Model file for the job. Use its own axes, mm. Face numbers are marked on the shaded views. Give positions to 0.01 mm unless a question says otherwise; leave off trailing zeros. Loops run counter-clockwise (first coordinate to the right, second up) from the corner with the lowest first, then second, coordinate; pieces in that order, holes last. Notation, with made-up numbers: M 45,25 L 88,25 A22 cw 88,52 Z; hole C 63,52 d2. An arc over 180 degrees is marked long. Answer in a Markdown table with one row per item.
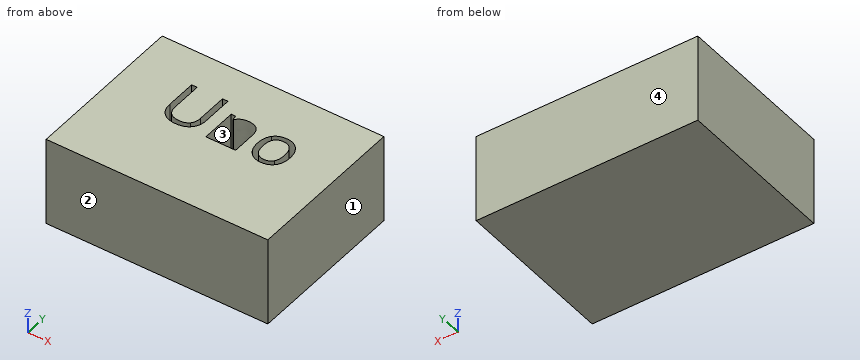
```python
from build123d import *

# Parameters (mm, degrees)
F0_W     = 75
F0_H     = 55
F1_DEPTH = 30
F3_DEPTH = 25


with BuildPart() as f1:
    # F0 (on Top) → F1 (new body)
    with BuildSketch(Plane.XY):
        with Locations((-1.7472282052, 5.8279882101)):
            Rectangle(F0_W, F0_H)
    extrude(amount=F1_DEPTH)

    # F2 (on face) → F3 (cut)
    with BuildSketch(Plane.XY.offset(30)):
        with BuildLine():
            Line((-4.0867042615, 16.8077548728), (-4.0867042615, 4.7675450332))
            Line((-4.0867042615, 4.7675450332), (-2.2622169894, 4.7675450332))
            Line((-2.2622169894, 4.7675450332), (-2.2622169894, 11.0847003856))
            add(Edge.make_bspline(
                [(-1.3833695559, 14.4577168355), (-2.2622169894, 13.4364961177), (-2.2622169894, 11.0847003856)],
                knots=[0, 0, 0, 1, 1, 1], degree=2))
            add(Edge.make_bspline(
                [(1.3832421649, 15.4789375533), (-0.5045221224, 15.4789375533), (-1.3833695559, 14.4577168355)],
                knots=[0, 0, 0, 1, 1, 1], degree=2))
            add(Edge.make_bspline(
                [(3.4836875311, 14.7530095732), (2.8140057867, 15.4789375533), (1.3832421649, 15.4789375533)],
                knots=[0, 0, 0, 1, 1, 1], degree=2))
            add(Edge.make_bspline(
                [(4.1533692754, 12.5576486842), (4.1533692754, 14.0270815931), (3.4836875311, 14.7530095732)],
                knots=[0, 0, 0, 1, 1, 1], degree=2))
            Line((4.1533692754, 12.5576486842), (4.1533692754, 4.7675450332))
            Line((4.1533692754, 4.7675450332), (5.9778565475, 4.7675450332))
            Line((5.9778565475, 4.7675450332), (5.9778565475, 12.6209256994))
            add(Edge.make_bspline(
                [(4.8792972555, 15.9798805904), (5.9778565475, 14.9305367547), (5.9778565475, 12.6209256994)],
                knots=[0, 0, 0, 1, 1, 1], degree=2))
            add(Edge.make_bspline(
                [(1.6047117181, 17.029224426), (3.7807379636, 17.029224426), (4.8792972555, 15.9798805904)],
                knots=[0, 0, 0, 1, 1, 1], degree=2))
            add(Edge.make_bspline(
                [(-0.6468954066, 16.5388275581), (0.363779142, 17.029224426), (1.6047117181, 17.029224426)],
                knots=[0, 0, 0, 1, 1, 1], degree=2))
            add(Edge.make_bspline(
                [(-2.2200323126, 15.1590370875), (-1.6575699552, 16.0484306902), (-0.6468954066, 16.5388275581)],
                knots=[0, 0, 0, 1, 1, 1], degree=2))
            Line((-2.2200323126, 15.1590370875), (-2.307917056, 15.1590370875))
            Line((-2.307917056, 15.1590370875), (-2.6032097937, 16.8077548728))
            Line((-2.6032097937, 16.8077548728), (-4.0867042615, 16.8077548728))
        make_face()
        with BuildLine():
            add(Edge.make_bspline(
                [(-12.2786519386, 4.7675450332), (-13.1925449458, 4.54607548), (-14.2813344906, 4.54607548)],
                knots=[0.6245807712, 0.6245807712, 0.6245807712, 1, 1, 1], degree=2))
            Line((-12.2786519386, 4.7675450332), (-16.2668224103, 4.7675450332))
            add(Edge.make_bspline(
                [(-14.2813344906, 4.54607548), (-15.3658863063, 4.54607548), (-16.2668224103, 4.7675450332)],
                knots=[0, 0, 0, 0.3739580419, 0.3739580419, 0.3739580419], degree=2))
        make_face()
        with BuildLine():
            Line((-16.2668224103, 4.7675450332), (-12.2786519386, 4.7675450332))
            add(Edge.make_bspline(
                [(-9.7218740054, 6.1174546912), (-10.7582183658, 5.1360014515), (-12.2786519386, 4.7675450332)],
                knots=[0, 0, 0, 0.6245807712, 0.6245807712, 0.6245807712], degree=2))
            add(Edge.make_bspline(
                [(-8.0626100508, 10.4378686745), (-8.0626100508, 7.6888339023), (-9.7218740054, 6.1174546912)],
                knots=[0, 0, 0, 1, 1, 1], degree=2))
            Line((-8.0626100508, 10.4378686745), (-8.0626100508, 20.8293607287))
            Line((-8.0626100508, 20.8293607287), (-9.9292819997, 20.8293607287))
            Line((-9.9292819997, 20.8293607287), (-9.9292819997, 10.3710762695))
            add(Edge.make_bspline(
                [(-11.0278412916, 7.2669871342), (-9.9292819997, 8.3497271724), (-9.9292819997, 10.3710762695)],
                knots=[0, 0, 0, 1, 1, 1], degree=2))
            add(Edge.make_bspline(
                [(-14.1582958499, 6.1842470961), (-12.1264005835, 6.1842470961), (-11.0278412916, 7.2669871342)],
                knots=[0, 0, 0, 1, 1, 1], degree=2))
            add(Edge.make_bspline(
                [(-17.3871813207, 7.2617140496), (-16.2886220288, 6.1842470961), (-14.1582958499, 6.1842470961)],
                knots=[0, 0, 0, 1, 1, 1], degree=2))
            add(Edge.make_bspline(
                [(-18.4857406127, 10.3499839311), (-18.4857406127, 8.3391810032), (-17.3871813207, 7.2617140496)],
                knots=[0, 0, 0, 1, 1, 1], degree=2))
            Line((-18.4857406127, 10.3499839311), (-18.4857406127, 20.8293607287))
            Line((-18.4857406127, 20.8293607287), (-20.3559279512, 20.8293607287))
            Line((-20.3559279512, 20.8293607287), (-20.3559279512, 10.4800533513))
            add(Edge.make_bspline(
                [(-18.7687294863, 6.1297585552), (-20.3559279512, 7.7134416305), (-20.3559279512, 10.4800533513)],
                knots=[0, 0, 0, 1, 1, 1], degree=2))
            add(Edge.make_bspline(
                [(-16.2668224103, 4.7675450332), (-17.7750766513, 5.1383065018), (-18.7687294863, 6.1297585552)],
                knots=[0.3739580419, 0.3739580419, 0.3739580419, 1, 1, 1], degree=2))
        make_face()
        with BuildLine():
            add(Edge.make_bspline(
                [(12.8943034011, 4.7675450332), (12.2413601129, 4.9561574078), (11.6657571374, 5.3053996626)],
                knots=[0.5400617249, 0.5400617249, 0.5400617249, 1, 1, 1], degree=2))
            Line((12.8943034011, 4.7675450332), (16.2966207559, 4.7675450332))
            add(Edge.make_bspline(
                [(18.6315018956, 6.2000663499), (17.691967628, 5.1513098305), (16.2966207559, 4.7675450332)],
                knots=[0, 0, 0, 0.6340763655, 0.6340763655, 0.6340763655], degree=2))
            add(Edge.make_bspline(
                [(20.1132386686, 10.7999538171), (20.1132386686, 7.8540572199), (18.6315018956, 6.2000663499)],
                knots=[0, 0, 0, 1, 1, 1], degree=2))
            add(Edge.make_bspline(
                [(18.6244711162, 15.3471104382), (20.1132386686, 13.6649964504), (20.1132386686, 10.7999538171)],
                knots=[0, 0, 0, 1, 1, 1], degree=2))
            add(Edge.make_bspline(
                [(14.6116537346, 17.029224426), (17.1357035637, 17.029224426), (18.6244711162, 15.3471104382)],
                knots=[0, 0, 0, 1, 1, 1], degree=2))
            add(Edge.make_bspline(
                [(10.5232554737, 15.3857797253), (11.9962037724, 17.029224426), (14.6116537346, 17.029224426)],
                knots=[0, 0, 0, 1, 1, 1], degree=2))
            add(Edge.make_bspline(
                [(9.0503071751, 10.7999538171), (9.0503071751, 13.7423350246), (10.5232554737, 15.3857797253)],
                knots=[0, 0, 0, 1, 1, 1], degree=2))
            add(Edge.make_bspline(
                [(9.7322927836, 7.481425908), (9.0503071751, 8.8981279709), (9.0503071751, 10.7999538171)],
                knots=[0, 0, 0, 1, 1, 1], degree=2))
            add(Edge.make_bspline(
                [(11.6657571374, 5.3053996626), (10.414278392, 6.0647238452), (9.7322927836, 7.481425908)],
                knots=[0, 0, 0, 1, 1, 1], degree=2))
        make_face()
        with BuildLine():
            add(Edge.make_bspline(
                [(10.9415868521, 10.7999538171), (10.9415868521, 8.4903427617), (11.8643766573, 7.282806388)],
                knots=[0, 0, 0, 1, 1, 1], degree=2))
            add(Edge.make_bspline(
                [(11.8538304881, 14.3030396872), (10.9415868521, 13.1271418211), (10.9415868521, 10.7999538171)],
                knots=[0, 0, 0, 1, 1, 1], degree=2))
            add(Edge.make_bspline(
                [(14.5554074988, 15.4789375533), (12.7660741242, 15.4789375533), (11.8538304881, 14.3030396872)],
                knots=[0, 0, 0, 1, 1, 1], degree=2))
            add(Edge.make_bspline(
                [(17.2974114915, 14.2872204334), (16.3693486017, 15.4789375533), (14.5554074988, 15.4789375533)],
                knots=[0, 0, 0, 1, 1, 1], degree=2))
            add(Edge.make_bspline(
                [(18.2254743813, 10.7999538171), (18.2254743813, 13.0955033135), (17.2974114915, 14.2872204334)],
                knots=[0, 0, 0, 1, 1, 1], degree=2))
            add(Edge.make_bspline(
                [(17.2974114915, 7.2775333034), (18.2254743813, 8.4797965925), (18.2254743813, 10.7999538171)],
                knots=[0, 0, 0, 1, 1, 1], degree=2))
            add(Edge.make_bspline(
                [(14.5764998373, 6.0752700144), (16.3693486017, 6.0752700144), (17.2974114915, 7.2775333034)],
                knots=[0, 0, 0, 1, 1, 1], degree=2))
            add(Edge.make_bspline(
                [(11.8643766573, 7.282806388), (12.7871664626, 6.0752700144), (14.5764998373, 6.0752700144)],
                knots=[0, 0, 0, 1, 1, 1], degree=2))
        make_face(mode=Mode.SUBTRACT)
        with BuildLine():
            Line((16.2966207559, 4.7675450332), (12.8943034011, 4.7675450332))
            add(Edge.make_bspline(
                [(14.5343151604, 4.54607548), (13.6609925365, 4.54607548), (12.8943034011, 4.7675450332)],
                knots=[0, 0, 0, 0.5400617249, 0.5400617249, 0.5400617249], degree=2))
            add(Edge.make_bspline(
                [(16.2966207559, 4.7675450332), (15.4913701164, 4.54607548), (14.5343151604, 4.54607548)],
                knots=[0.6340763655, 0.6340763655, 0.6340763655, 1, 1, 1], degree=2))
        make_face()
        with BuildLine():
            Line((-2.2622169894, 11.0847003856), (-2.2622169894, 4.7675450332))
            Line((-2.2622169894, 4.7675450332), (4.1533692754, 4.7675450332))
            Line((4.1533692754, 4.7675450332), (4.1533692754, 12.5576486842))
            add(Edge.make_bspline(
                [(4.1533692754, 12.5576486842), (4.1533692754, 14.0270815931), (3.4836875311, 14.7530095732)],
                knots=[0, 0, 0, 1, 1, 1], degree=2))
            add(Edge.make_bspline(
                [(3.4836875311, 14.7530095732), (2.8140057867, 15.4789375533), (1.3832421649, 15.4789375533)],
                knots=[0, 0, 0, 1, 1, 1], degree=2))
            add(Edge.make_bspline(
                [(1.3832421649, 15.4789375533), (-0.5045221224, 15.4789375533), (-1.3833695559, 14.4577168355)],
                knots=[0, 0, 0, 1, 1, 1], degree=2))
            add(Edge.make_bspline(
                [(-1.3833695559, 14.4577168355), (-2.2622169894, 13.4364961177), (-2.2622169894, 11.0847003856)],
                knots=[0, 0, 0, 1, 1, 1], degree=2))
        make_face()
    extrude(amount=-F3_DEPTH, mode=Mode.SUBTRACT)


solid = f1.part
```
Q1. Saw through at B-B (y = 19.5). Give the cut face in (x, z).
Reported:
| item | result |
|---|---|
| outline | M -39.25,0 L 35.75,0 L 35.75,30 L -8.06,30 L -8.06,5 L -9.93,5 L -9.93,30 L -18.49,30 L -18.49,5 L -20.36,5 L -20.36,30 L -39.25,30 Z |
Q2. Saw through at A-A (z = 13.5). Give the number of separate pieces and of enclosed holes in the cut face, and give its area (3 significant figures).
Reported:
| item | result |
|---|---|
| separate pieces | 2 |
| enclosed holes | 3 |
| area | 3,880 mm² |
Q3. Probe probe 1 along Y at (x, z) = (17, 6); probe 2 along Y at (x, z) = (16, 16); probe 3 along Y at (x, z) = (-4, 21). List the from-to ranges inside material, lowest first.
Reported:
| item | result |
|---|---|
| probe 1 | -21.67 to 5.02, 6.94 to 14.62, 16.56 to 33.33 |
| probe 2 | -21.67 to 4.69, 6.31 to 15.24, 16.89 to 33.33 |
| probe 3 | -21.67 to 4.77, 16.81 to 33.33 |
Q4. Mould opens along Y. For the marked faces 1, 2, 3 and 4 say: released by +Y, released by -Y, zero draft, split by the parting line, or undercut.
Reported:
| item | result |
|---|---|
| face 1 | zero draft |
| face 2 | released by -Y |
| face 3 | undercut |
| face 4 | released by +Y |
Q5. Drop a flat-ended pin along its axis: pin 1 (5 mm diameter, centred on x = -1.5, y = 8.5, fed in from +Z). Give the stop position or say it passes through.
Reported:
| item | result |
|---|---|
| pin 1 | z = 5 |
